Build history of the part. All positions in model axes, mm. Face numbers are marked on the shaded views. A direction names the side the tool comes from. Coordinates: 2 decimals unless noted, no trailing zeros. Order: outer loops, then holes, each group sorted by start corner. A loop starts at its lowest first (then second) coordinate and runs counter-clockwise, first axis right, second up. Notation, with made-up numbers: (-14.5, -35) - (-1.5, -35) arc R21 cw to (-1.5, -22) - close; hole circle Ø9 at (84.5, -4). An arc over 180 degrees is marked (long way). Write each question's results on one line, items separated by ' | '.
from build123d import *

# Parameters (mm, degrees)
SKETCH10_R         = 11.5
CUT_EXTRUDE1_DEPTH = 70
SKETCH12_R         = 15
CUT_EXTRUDE2_DEPTH = 4
CIRPATTERN1_COUNT  = 4


with BuildPart() as part:
    # Sketch1 → Revolve1 (revolve)
    with BuildSketch(Plane.XY):
        Polygon((37, 43.55415604), (48.996866339, 43.55415604), (48.996866339, 36), (45, 36), (45, 34), (49, 34), (49, 31), (45, 31), (45, 29), (49, 29), (49, 26), (45, 26), (45, 23), (49, 23), (49, -43), (42, -43), (42, -40), (45, -40), (45, -29.408174518), (20, -25), (20, 9), (39, 12.350212633), (39, 20), (0, 20), (0, 35.55415604), (37, 31.55415604), align=None)
    revolve(axis=Axis((0, 43, 0), (0, 1, 0)))

    # Sketch10 → Cut-Extrude1 (cut, symmetric)
    with BuildSketch(Plane(origin=(0, 0, 0), x_dir=(0, 0, -1), z_dir=(1, 0, 0))):
        with Locations((0, -8)):
            Circle(SKETCH10_R)
    extrude(amount=CUT_EXTRUDE1_DEPTH, both=True, mode=Mode.SUBTRACT)

    # Sketch12 → Cut-Extrude2 (cut)
    with BuildSketch(Plane(origin=(0, 43.55415604, 0), x_dir=(1, 0, 0), z_dir=(0, 1, 0))):
        with Locations((-21.213203436, 21.213203436)):
            Circle(SKETCH12_R)
    cut_extrude2 = extrude(amount=-CUT_EXTRUDE2_DEPTH, mode=Mode.SUBTRACT)

    # CirPattern1: Cut-Extrude2 ×4 about axis
    cirpattern1_axis = Axis((0, 0, 0), (0, 1, 0))
    for i in range(1, CIRPATTERN1_COUNT):
        add(cut_extrude2.rotate(cirpattern1_axis, i * 360 / CIRPATTERN1_COUNT), mode=Mode.SUBTRACT)


solid = part.part
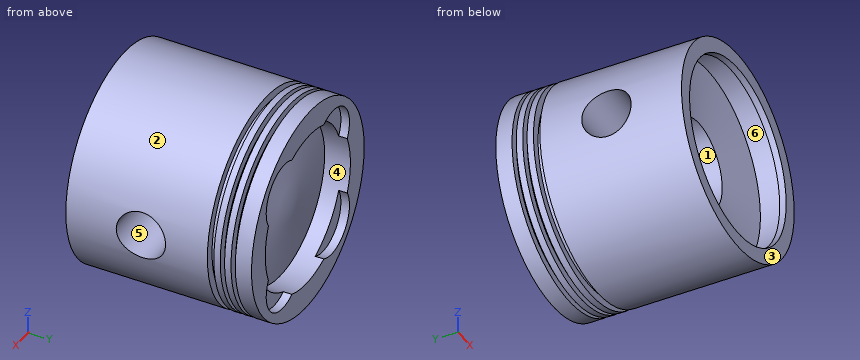
1. Tool access for the marked faces 4, 5 and 6: list every direction of +Z, -Z, +X, -X, +Y, -Y with a clear straight run to the whole face (end or side of a thin tool).
Solved:
face 4: +Y | face 5: +X, -X | face 6: none
2. Band-saw the part on D-D on y = -35. Give the cut face in (x, z), then the cut area to 3 significant figures.
Solved:
outline: circle Ø98 at (0, 0); hole circle Ø90 at (0, 0) | area: 1,180 mm2
3. Band-saw the part on C-C on x = 25. Give the number of separate pieces and of enclosed holes in the cut face, then the cut area to 3 significant figures.
Solved:
separate pieces: 1 | enclosed holes: 2 | area: 4,420 mm2
4. Two-plate mould, pull along Z, no slides. Class the marked faces 1, 2 and 3: +Z half, -Z half, draft (parallel to the pull), parting line (faces both ways), or undercut.
Solved:
face 1: undercut | face 2: parting line | face 3: draft
5. Drop flat-ended pins along their axis: pin 1 Ø1 at (x, z) = (-36.5, -13.5) entering from -Y; pin 2 Ø12 at (y, z) = (-11, -18) entering from +X; pin 3 Ø1.5 at (x, z) = (-6, -6.5) entering from +Y. Give the stop position or say it passes through.
Solved:
pin 1: stops at y = -28.42 | pin 2: stops at x = 47.51 | pin 3: stops at y = 34.68
6. Band-saw the part on B-B on y = 6.5. Give the cut face in (x, z).
Solved:
outline: circle Ø98 at (0, 0); hole circle Ø40 at (0, 0)
7. Band-saw the part on A-A on y = -8. Give the cut face in (x, z).
Solved:
outline: (-47.63, -11.5) arc R49 ccw to (47.63, -11.5) - (16.36, -11.5) arc R20 cw to (-16.36, -11.5) - close; (-47.63, 11.5) - (-16.36, 11.5) arc R20 cw to (16.36, 11.5) - (47.63, 11.5) arc R49 ccw to start
8. Probe line 1 (Y direction, x = 24, z = 38.5); line 2 (Z direction, x = 0, y = -33); line 3 (X direction, y = -42, z = 0). List the from-to ranges inside material, lowest first.
Solved:
line 1: y = -43 to 23, 26 to 29, 31 to 34, 36 to 43.55 | line 2: z = -49 to -45, 45 to 49 | line 3: x = -49 to -42, 42 to 49
